Build history of the part. All positions in model axes, mm. A direction names the side the tool comes from. Round coordinates to 2 decimals unless told otherwise and drop trailing zeros. Write each loop counter-clockwise with the first axis right and the second up, starting at its lowest first coordinate (ties: lowest second). Pieces come first, ordered by that corner, then holes. Notation, with made-up numbers: M 88,77.5 L 110,77.5 A25 ccw 110,101.5 Z; hole C 19,52.25 d2. An arc over 180 degrees is marked long. Use a Markdown table: item, result.
from build123d import *

# Parameters (mm, degrees)
SKETCH2_W           = 60
SKETCH2_H           = 36
BOSS_EXTRUDE2_DEPTH = 15
SKETCH5_W           = 55
SKETCH5_H           = 31
CUT_EXTRUDE1_DEPTH  = 12.5
SKETCH6_W           = 6
SKETCH6_H           = 6
SKETCH6_R           = 1.75
BOSS_EXTRUDE3_DEPTH = 2.5
SKETCH7_R           = 6
CUT_EXTRUDE2_DEPTH  = 15
BOSS_EXTRUDE4_DEPTH = 12.5
SKETCH10_W          = 8
SKETCH10_H          = 8
CUT_EXTRUDE3_DEPTH  = 12.5


with BuildPart() as part:
    # Sketch2 → Boss-Extrude2 (new body)
    with BuildSketch(Plane(origin=(0, 0, 0), x_dir=(1, 0, 0), z_dir=(0, 1, 0))):
        Rectangle(SKETCH2_W, SKETCH2_H)
    extrude(amount=BOSS_EXTRUDE2_DEPTH)

    # Sketch5 → Cut-Extrude1 (cut)
    with BuildSketch(Plane(origin=(0, 0, 0), x_dir=(1, 0, 0), z_dir=(0, 1, 0))):
        Rectangle(SKETCH5_W, SKETCH5_H)
    extrude(amount=CUT_EXTRUDE1_DEPTH, mode=Mode.SUBTRACT)

    # Sketch6 → Boss-Extrude3 (add)
    with BuildSketch(Plane(origin=(0, 0, 0), x_dir=(1, 0, 0), z_dir=(0, 1, 0))):
        with Locations((-33, 15)):
            Rectangle(SKETCH6_W, SKETCH6_H)
        with Locations(Location((-33, 15, 0), (0, 0, 270))):  # turned: the seam where the file's is
            Circle(SKETCH6_R, mode=Mode.SUBTRACT)
        with Locations((33, -14.5)):
            Rectangle(SKETCH6_W, SKETCH6_H)
        with Locations(Location((33, -14.5, 0), (0, 0, 270))):  # turned: the seam where the file's is
            Circle(SKETCH6_R, mode=Mode.SUBTRACT)
    extrude(amount=BOSS_EXTRUDE3_DEPTH)

    # Sketch7 → Cut-Extrude2 (cut)
    with BuildSketch(Plane(origin=(0, 0, 0), x_dir=(1, 0, 0), z_dir=(0, 1, 0))):
        with Locations(Location((5.404735112, 8.226712099, 0), (0, 0, 270))):  # turned: the seam where the file's is
            Circle(SKETCH7_R)
    extrude(amount=CUT_EXTRUDE2_DEPTH, mode=Mode.SUBTRACT)

    # Sketch8 → Boss-Extrude4 (add)
    with BuildSketch(Plane(origin=(0, 0, 0), x_dir=(1, 0, 0), z_dir=(0, 1, 0))):
        Polygon((-21.035533906, 0), (-17.5, 0), (-17.5, 2.5), (-14.447985549, 2.5), (-14.447985549, 6.535533906), (-21.035533906, 6.535533906), align=None)
    extrude(amount=BOSS_EXTRUDE4_DEPTH)

    # Sketch10 → Cut-Extrude3 (cut)
    with BuildSketch(Plane(origin=(30, 0, 0), x_dir=(0, 0, -1), z_dir=(1, 0, 0))):
        with Locations((10.327095022, 4)):
            Rectangle(SKETCH10_W, SKETCH10_H)
    extrude(amount=-CUT_EXTRUDE3_DEPTH, mode=Mode.SUBTRACT)


solid = part.part
Q1. Drill centre lines: L1, parallel to X at y = 1.05, z = 14.5; L2, parallel to X at y = 0.8, z = -15; L3, parallel to Z at x = -17, y = 2.75. Where is each one in solid material? Low to high.
Response values:
| item | result |
|---|---|
| L1 | x = -30 to -27.5, 27.5 to 31.25, 34.75 to 36 |
| L2 | x = -36 to -34.75, -31.25 to -27.5, 27.5 to 30 |
| L3 | z = -18 to -15.5, -6.54 to -2.5, 15.5 to 18 |
Q2. Cut at A-A on y = 4.5. Give the cut face in (x, z), and give its area (3 significant figures).
Response values:
| item | result |
|---|---|
| outline | M -30,-18 L 30,-18 L 30,-14.33 L 27.5,-14.33 L 27.5,-15.5 L -27.5,-15.5 L -27.5,15.5 L 27.5,15.5 L 27.5,-6.33 L 30,-6.33 L 30,18 L -30,18 Z; M -21.04,-6.54 L -14.45,-6.54 L -14.45,-2.5 L -17.5,-2.5 L -17.5,0 L -21.04,0 Z |
| area | 470 mm2 |
Q3. Two-plate mould, pull along Z, no slides. Class faces 4 (the flat face through (29, 8, -10)), 5 (the flat face through (-14.448, 6, -4)), 6 (the flat face through (0, 7, 18)), 7 (the flat face through (36, 1, 15)): +Z half, -Z half, draft (parallel to the pull), parting line (faces both ways), or undercut.
Response values:
| item | result |
|---|---|
| face 4 | undercut |
| face 5 | undercut |
| face 6 | +Z half |
| face 7 | draft |
Q4. Which spindle directions (+Z, -Z, +X, -X, +Y, -Y) get a long thin tool onto all of the face, cutting with end or side? Do faces 1 (the flat face through (-31.7, 2.5, -16.4)), 2 (the flat face through (-33, 1, -12)), 3 (the flat face through (-27.5, 6, 0)). Say none if no direction does.
Response values:
| item | result |
|---|---|
| face 1 | +Z, -Z, -X, +Y |
| face 2 | +Z, -X, +Y, -Y |
| face 3 | -Y |
Q5. Drop flat-ended pins along their axis: P1, Ø14, axis at x = 5.4, z = -8.23, coming from the -Y side; P2, Ø7.5, axis at y = 8.5, z = -3.5, coming from the +X side; P3, Ø1.2, axis at x = 33, y = 1.5, coming from the +Z side; P4, Ø3, axis at x = -33, z = -15, coming from the +Y side. Give the stop position or say it passes through.
Response values:
| item | result |
|---|---|
| P1 | stops at y = 12.5 |
| P2 | stops at x = 30 |
| P3 | stops at z = 17.5 |
| P4 | passes through |
Q6. Cut at C-C on y = 1. Give the cut face in (x, z).
Response values:
| item | result |
|---|---|
| outline | M -36,-18 L 30,-18 L 30,-14.33 L 27.5,-14.33 L 27.5,-15.5 L -27.5,-15.5 L -27.5,15.5 L 27.5,15.5 L 27.5,-6.33 L 30,-6.33 L 30,11.5 L 36,11.5 L 36,17.5 L 30,17.5 L 30,18 L -30,18 L -30,-12 L -36,-12 Z; M -21.04,-6.54 L -14.45,-6.54 L -14.45,-2.5 L -17.5,-2.5 L -17.5,0 L -21.04,0 Z; hole C -33,-15 d3.5; hole C 33,14.5 d3.5 |
Q7. Cut at D-D on z = 14.5. Give the cut face in (x, y).
Response values:
| item | result |
|---|---|
| outline | M -30,0 L -27.5,0 L -27.5,12.5 L 27.5,12.5 L 27.5,0 L 31.25,0 L 31.25,2.5 L 30,2.5 L 30,15 L -30,15 Z; M 34.75,0 L 36,0 L 36,2.5 L 34.75,2.5 Z |
Q8. Cut at B-B on x = 33. Give the cut face in (y, z).
Response values:
| item | result |
|---|---|
| outline | M 0,11.5 L 2.5,11.5 L 2.5,12.75 L 0,12.75 Z; M 0,16.25 L 2.5,16.25 L 2.5,17.5 L 0,17.5 Z |
